CAD build for the part. Positions are in the model's coordinates, mm. Give positions to 0.01 mm unless a question says otherwise; leave off trailing zeros. Write each loop counter-clockwise with the first axis right and the second up, starting at its lowest first coordinate (ties: lowest second). Pieces come first, ordered by that corner, then holes. Notation, with made-up numbers: (43, 75.5) -> (83, 75.5) arc R22 ccw to (83, 108.5) -> close; hole circle Ø7 at (21.5, 10). An arc over 180 degrees is marked (long way). Answer as a JSON object with one key per item and string values.
```python
from build123d import *

# Parameters (mm, degrees)
BOSS_EXTRUDE1_DEPTH = 127
FILLET3_R           = 10
FILLET4_R           = 5.08


with BuildPart() as part:
    # Sketch1 → Boss-Extrude1 (new body)
    with BuildSketch(Plane(origin=(0, 0, 0), x_dir=(0, 0, -1), z_dir=(1, 0, 0))):
        Polygon((-4.750453706, 0), (-2.375226853, 12.992673374), (0, 0), (10.362546294, 0), (10.362546294, 25.4), (-15.037453706, 25.4), (-15.037453706, 0), align=None)
    extrude(amount=BOSS_EXTRUDE1_DEPTH)

    # Fillet3
    fillet3_edges = [part.edges().sort_by_distance(p)[0] for p in [
        (63.5, 25.4, 15.037453706),
        (63.5, 25.4, -10.362546294),
    ]]
    fillet(fillet3_edges, radius=FILLET3_R)

    # Fillet4
    fillet4_edges = [part.edges().sort_by_distance(p)[0] for p in [
        (0, 25.4, 2.337453706),
        (0, 7.7, -10.362546294),
        (0, 22.471067812, -7.433614106),
        (0, 22.471067812, 12.108521518),
        (127, 25.4, 2.337453706),
        (127, 7.7, -10.362546294),
        (127, 22.471067812, -7.433614106),
        (127, 22.471067812, 12.108521518),
        (127, 7.7, 15.037453706),
        (0, 7.7, 15.037453706),
    ]]
    fillet(fillet4_edges, radius=FILLET4_R)


solid = part.part
```
1) Slice it at B-B (y = 7.25). List the corners of the cut face in (x, z), then the cut area to 3 significant figures.
Model answer:
{"outline": "(0, -5.28) arc R5.08 ccw to (5.08, -10.36) -> (121.92, -10.36) arc R5.08 ccw to (127, -5.28) -> (127, 1.33) -> (0, 1.33) -> close; (0, 3.43) -> (127, 3.43) -> (127, 9.96) arc R5.08 ccw to (121.92, 15.04) -> (5.08, 15.04) arc R5.08 ccw to (0, 9.96) -> close", "area": "2,940 mm2"}
2) Pin check, flat tips, straight feed: pin 1 (3 mm diameter, centred on x = 48, z = 7, fed in from -Y); pin 2 (2 mm diameter, centred on x = 17.5, z = -3, fed in from +Y) (3 decimals); pin 3 (2 mm diameter, centred on x = 56, z = 12, fed in from +Y). Stop position of each tip, or through.
Model answer:
{"pin 1": "stops at y = 0", "pin 2": "stops at y = 25.265", "pin 3": "stops at y = 23.43"}
3) Wall check: probe 1 along X at (y, z) = (5.5, -5.5); probe 2 along Y at (x, z) = (41.5, 13.75); probe 3 along Z at (x, y) = (78.5, 4). Give the ranges that are in metal, low to high.
Model answer:
{"probe 1": "x = 0 to 127", "probe 2": "y = 0 to 20.31", "probe 3": "z = -10.36 to 0.73, 4.02 to 15.04"}
4) Slice it at A-A (x = 46). List the corners of the cut face in (y, z), then the cut area to 3 significant figures.
Model answer:
{"outline": "(0, -10.36) -> (15.4, -10.36) arc R10 ccw to (25.4, -0.36) -> (25.4, 5.04) arc R10 ccw to (15.4, 15.04) -> (0, 15.04) -> (0, 4.75) -> (12.99, 2.38) -> (0, 0) -> close", "area": "571 mm2"}
5) Mould opens along Z. For faces 1 (the cylindrical face through (125.551, 7.808, -8.835)), 2 (the flat face through (0, 10, 4)), 3 (the flat face through (62.611, 6.587, 1.204)) say: released by +Z, released by -Z, zero draft, split by the parting line, or undercut.
Model answer:
{"face 1": "released by -Z", "face 2": "zero draft", "face 3": "undercut"}
